The listing builds one solid part. Answer for the finished solid, in the listing's coordinates (mm). A direction names the side the tool comes from. Give positions to 0.01 mm unless a question says otherwise; leave off trailing zeros. Order: outer loops, then holes, each group sorted by start corner. A loop starts at its lowest first (then second) coordinate and runs counter-clockwise, first axis right, second up. Notation, with made-up numbers: (78, 7) -> (122, 7) arc R22 ccw to (122, 35) -> close; hole circle Ø7 at (-18, 9.25). An arc over 180 degrees is marked (long way). Write item = value, one per line. Start each with the question number.
```python
from build123d import *

# Parameters (mm, degrees)
SKETCH2_W           = 88.9
SKETCH2_H           = 25.4
SKETCH2_R           = 3.175
BOSS_EXTRUDE1_DEPTH = 6.35
SKETCH3_R           = 5.08
CUT_EXTRUDE1_DEPTH  = 93.675198948
SKETCH4_R           = 5.08
SKETCH4_R_2         = 3.175
BOSS_EXTRUDE2_DEPTH = 22.225


with BuildPart() as part:
    # Sketch2 → Boss-Extrude1 (new body)
    with BuildSketch(Plane(origin=(0, 0, 0), x_dir=(1, 0, 0), z_dir=(0, 1, 0))):
        with Locations((0, 12.7)):
            Rectangle(SKETCH2_W, SKETCH2_H)
        with Locations(Location((-31.75, 12.7, 0), (0, 0, 270))):
            Circle(SKETCH2_R, mode=Mode.SUBTRACT)
        with Locations(Location((0, 12.7, 0), (0, 0, 270))):
            Circle(SKETCH2_R, mode=Mode.SUBTRACT)
        with Locations(Location((31.75, 12.7, 0), (0, 0, 270))):
            Circle(SKETCH2_R, mode=Mode.SUBTRACT)
    extrude(amount=BOSS_EXTRUDE1_DEPTH)

    # Sketch3 → Cut-Extrude1 (cut, through all)
    with BuildSketch(Plane.ZY.offset(44.45)):
        with Locations((0, 6.35)):
            Circle(SKETCH3_R)
    extrude(amount=-CUT_EXTRUDE1_DEPTH, mode=Mode.SUBTRACT)

    # Sketch4 → Boss-Extrude2 (add)
    with BuildSketch(Plane(origin=(9.525, 0, 0), x_dir=(0, 0, -1), z_dir=(1, 0, 0))):
        with Locations((0, 6.35)):
            Circle(SKETCH4_R)
        with Locations((0, 6.35)):
            Circle(SKETCH4_R_2, mode=Mode.SUBTRACT)
    boss_extrude2 = extrude(amount=BOSS_EXTRUDE2_DEPTH)

    # Mirror1: Boss-Extrude2 across plane
    add(boss_extrude2.mirror(Plane(origin=(0, 0, 0), x_dir=(0, 0, 1), z_dir=(1, 0, 0))))


solid = part.part
```
Item 1: A cutting plane is placed at A-A, the plane x = 0. Write down the section's boundary in (y, z) (3 decimals), plus the area to 3 significant figures.
Item 2: Flat-ended cylindrical pins translate along their axes: pin 1 (8.5 mm diameter, centred on x = 0, z = -12.7, fed in from +Y); pin 2 (1.4 mm diameter, centred on x = -19, y = 1, fed in from +Z); pin 3 (1 mm diameter, centred on x = 35, z = 2, fed in from -Y); pin 4 (5 mm diameter, centred on y = 8.5, z = -0.5, fed in from +X). Find the tip coordinate at first contact, or state that the pin passes through.
Item 3: The mould has two halves that part along Y. Classify faces 1 (the flat face through (-1, 0, -19)), 2 (the flat face through (9.525, 3, 0)), 3 (the cylindrical face through (20.482, 9.027, -1.707)): +Y half, -Y half, draft (parallel to the pull), parting line (faces both ways), or undercut.
Item 4: A cutting plane is placed at D-D, the plane x = -11. Write down the section's boundary in (y, z) (3 decimals), plus the area to 3 significant figures.
Item 5: Consider L1, parallel to X at y = 4, z = -12.7 (3 decimals); L2, parallel to Z at x = 30.5, y = 5; L3, parallel to X at y = 1.75, z = -1 (3 decimals). Determine where each line is inside the solid, lowest interval first. Write a range as from..to.
Item 6: A cutting plane is placed at C-C, the plane x = 30. Write down the section's boundary in (y, z) (3 decimals).
Item 7: Which of the six approach directions +Z, -Z, +X, -X, +Y, -Y give full straight-line access (tool end or side, diameter ignored) to faces 4 (the cylindrical face through (20.48, 10.06, 3.47)), 5 (the flat face through (-31.75, 3, 0)), 6 (the cylindrical face through (-0.133, 2.798, -3.631)), 7 (the flat face through (-1, 6.35, -18)), 8 (the flat face through (31.75, 3, 0))?
Item 8: A cutting plane is placed at B-B, the plane y = 7.5. Write down the section's boundary in (x, z) (3 decimals).
Check values:
q1.outline = (0, -25.4) -> (6.35, -25.4) -> (6.35, -15.875) -> (0, -15.875) -> close; (0, -9.525) -> (6.35, -9.525) -> (6.35, -5.08) arc R5.08 cw to (1.27, 0) -> (0, 0) -> close
q1.area = 101 mm^2
q2.pin_1 = 6.35
q2.pin_2 = 2.05
q2.pin_3 = through
q2.pin_4 = 31.75
q3.face_1 = -Y half
q3.face_2 = draft
q3.face_3 = undercut
q4.outline = (0, -25.4) -> (6.35, -25.4) -> (6.35, -5.08) arc R5.08 ccw (long way) to (1.27, 0) -> (0, 0) -> close; hole circle Ø6.35 at (6.35, 0)
q4.area = 190 mm^2
q5.L1 = -44.45..-34.925, -28.575..-3.175, 3.175..28.575, 34.925..44.45
q5.L2 = -25.4..-15.62, -9.78..-2.87, 2.87..4.9
q5.L3 = -31.75..-9.525, 9.525..31.75
q6.outline = (0, -25.4) -> (6.35, -25.4) -> (6.35, -15.349) -> (0, -15.349) -> close; (0, -10.051) -> (6.35, -10.051) -> (6.35, -5.08) arc R5.08 ccw (long way) to (1.27, 0) -> (0, 0) -> close; hole circle Ø6.35 at (6.35, 0)
q7.face_4 = +X, -X
q7.face_5 = +Z, -X, +Y
q7.face_6 = +Z, +Y
q7.face_7 = -Z, +X, -X, +Y
q7.face_8 = +Z, +X, +Y
q8.outline = (-31.75, -4.948) -> (-9.525, -4.948) -> (-9.525, -2.959) -> (-31.75, -2.959) -> close; (-31.75, 2.959) -> (-9.525, 2.959) -> (-9.525, 4.948) -> (-31.75, 4.948) -> close; (9.525, -4.948) -> (31.75, -4.948) -> (31.75, -2.959) -> (9.525, -2.959) -> close; (9.525, 2.959) -> (31.75, 2.959) -> (31.75, 4.948) -> (9.525, 4.948) -> close
